The figure shows three views and two pictorial views of one solid part (mm, origin at its lowest corner). Answer the questions. Give positions to 0.01 mm unless a question says otherwise; leave off trailing zeros. Loops run counter-clockwise (first coordinate to the right, second up) from the corner with the lowest first, then second, coordinate; pieces in that order, holes last. Notation, with made-up numbers: M 39,-26.75 L 82,-26.75 A23 ccw 82,-7.75 Z; hole C 40.25,66.25 d6. An arc over 180 degrees is marked long. Write item = value, one per line. Start each with the question number.
1. Section C-C on x = 11 is taken. Determine the outline of the cut face in (y, z) (1 decimal).
2. Section B-B on y = 13.75 is taken. Determine the outline of the cut face in (x, z) (1 decimal).
3. Flat-ended cylindrical pins translate along their axes: pin 1 Ø1.5 at (x, z) = (9, 30) entering from -Y; pin 2 Ø2 at (x, z) = (11, 54) entering from -Y. Find the tip coordinate at first contact, or state that the pin passes through.
4. Consider L1, parallel to Y at x = 7.5, z = 65 (1 decimal); L2, parallel to X at y = 7.75, z = 12; L3, parallel to X at y = 0.5, z = 66 (1 decimal). Determine where each line is inside the solid, lowest interval first. Write a range as [from, to].
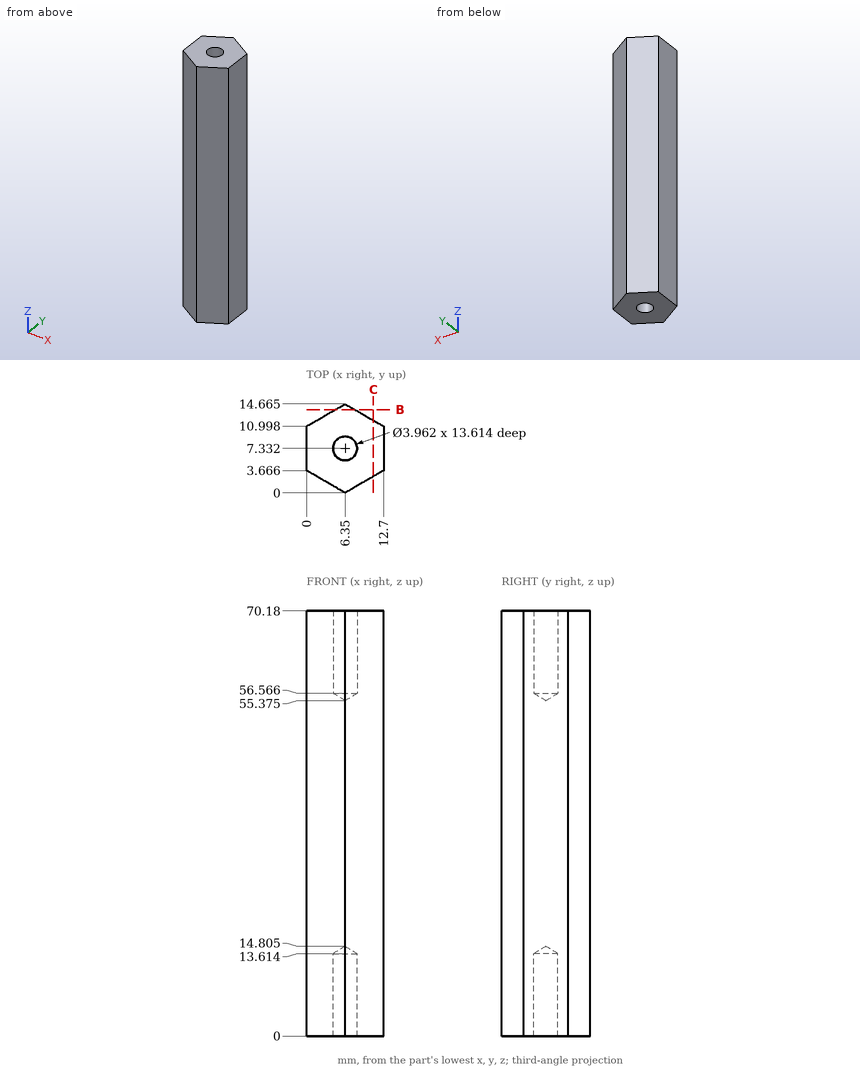
Verdict:
q1.outline = M 2.7,0 L 12,0 L 12,70.2 L 2.7,70.2 Z
q2.outline = M 4.8,0 L 7.9,0 L 7.9,70.2 L 4.8,70.2 Z
q3.pin_1 = 1.1
q3.pin_2 = 2.11
q4.L1 = [0.7, 5.7], [8.9, 14]
q4.L2 = [0, 4.41], [8.29, 12.7]
q4.L3 = [5.5, 7.2]
